The listing builds one solid part. Answer for the finished solid, in the listing's coordinates (mm). A direction names the side the tool comes from. Coordinates: 2 decimals unless noted, no trailing zeros. Order: outer loops, then holes, each group sorted by start corner. A loop starts at its lowest first (then second) coordinate and runs counter-clockwise, first axis right, second up. Notation, with made-up numbers: (-0.5, 26) -> (46.5, 26) arc R18 ccw to (46.5, 30) -> close; hole circle Ø10 at (38.5, 50). An arc over 180 degrees is marked (long way). One line per question, with ' | ' between items.
from build123d import *

# Parameters (mm, degrees)
SKETCH_1_R          = 39
EXTRUDE_1_DEPTH     = 4
SKETCH_3_R          = 37
EXTRUDE_2_DEPTH     = 8
SKETCH_4_R          = 36
EXTRUDE_3_DEPTH     = 8
SKETCH_5_W          = 3
SKETCH_5_H          = 1.5
SKETCH_7_R          = 27
CUT_EXTRUDE_1_DEPTH = 17
CHAMFER_2_SIZE      = 1
SKETCH_14_R         = 1.3
CUT_EXTRUDE_4_DEPTH = 7
CUT_EXTRUDE_START   = 7
SKETCH_16_R         = 1.3
CUT_EXTRUDE_5_DEPTH = 7
SKETCH_18_R         = 1.3
CUT_EXTRUDE_6_DEPTH = 7
CHAMFER_3_SIZE      = 1


with BuildPart() as part:
    # Sketch 1 → Бобышка-Вытянуть1 (new body)
    with BuildSketch(Plane.XY):
        Circle(SKETCH_1_R)
    extrude(amount=EXTRUDE_1_DEPTH)

    # Эскиз3 → Бобышка-Вытянуть2 (add)
    with BuildSketch(Plane(origin=(0, 0, 0), x_dir=(-1, 0, 0), z_dir=(0, 0, -1))):
        with Locations(Location((0, 0, 0), (0, 0, 180))):
            Circle(SKETCH_3_R)
    extrude(amount=EXTRUDE_2_DEPTH)

    # Эскиз4 → Бобышка-Вытянуть3 (add)
    with BuildSketch(Plane(origin=(0, 0, -8), x_dir=(-1, 0, 0), z_dir=(0, 0, -1))):
        Circle(SKETCH_4_R)
    extrude(amount=EXTRUDE_3_DEPTH)

    # Эскиз5 → Вырез-Повернуть1 (revolve, cut)
    with BuildSketch(Plane(origin=(0, 0, 0), x_dir=(0, 0, -1), z_dir=(1, 0, 0)), mode=Mode.PRIVATE) as cut_revolve_1_sk:
        with Locations((12.5, 35.25)):
            Rectangle(SKETCH_5_W, SKETCH_5_H)
    revolve(cut_revolve_1_sk.sketch.rotate(Axis((0, 0, 46.650977883), (0, 0, -1)), 90), axis=Axis((0, 0, 46.650977883), (0, 0, -1)), mode=Mode.SUBTRACT)

    # Эскиз7 → Вырез-Вытянуть1 (cut)
    with BuildSketch(Plane(origin=(0, 0, -16), x_dir=(-1, 0, 0), z_dir=(0, 0, -1))):
        Circle(SKETCH_7_R)
    extrude(amount=-CUT_EXTRUDE_1_DEPTH, mode=Mode.SUBTRACT)

    # Фаска2
    chamfer_2_edges = [part.edges().sort_by_distance(p)[0] for p in [
        (36, 0, -16),
    ]]
    chamfer(chamfer_2_edges, length=CHAMFER_2_SIZE)

    # Эскиз14 → Вырез-Вытянуть4 (cut)
    with BuildSketch(Plane(origin=(37, 0, 0), x_dir=(0, 0, -1), z_dir=(1, 0, 0))):
        with Locations((5, 0)):
            Circle(SKETCH_14_R)
    extrude(amount=-CUT_EXTRUDE_4_DEPTH, mode=Mode.SUBTRACT)

    # Эскиз16 → Вырез-Вытянуть5 (cut)
    with BuildSketch(Plane(origin=(-37, 0, 0), x_dir=(0, 0, -1), z_dir=(1, 0, 0)).offset(CUT_EXTRUDE_START)):
        with Locations((5, 0)):
            Circle(SKETCH_16_R)
    extrude(amount=-CUT_EXTRUDE_5_DEPTH, mode=Mode.SUBTRACT)

    # Эскиз18 → Вырез-Вытянуть6 (cut)
    with BuildSketch(Plane.XY.offset(4)):
        with Locations((6.5, 32.5)):
            Circle(SKETCH_18_R)
        with Locations(Location((-6.5, 32.5, 0), (0, 0, 180))):
            Circle(SKETCH_18_R)
        with Locations(Location((6.5, -32.5, 0), (0, 0, 180))):
            Circle(SKETCH_18_R)
        with Locations((-6.5, -32.5)):
            Circle(SKETCH_18_R)
    extrude(amount=-CUT_EXTRUDE_6_DEPTH, mode=Mode.SUBTRACT)

    # Фаска3
    chamfer_3_edges = [part.edges().sort_by_distance(p)[0] for p in [
        (27, 0, 1),
        (27, 0, -16),
        (-39, 0, 4),
    ]]
    chamfer(chamfer_3_edges, length=CHAMFER_3_SIZE)


solid = part.part
Item 1: Section A-A, the plane z = -9 is taken. Give the vertices of the cut face in (x, y), plus the area to 3 significant figures.
Computed values:
outline: circle Ø72 at (0, 0); hole circle Ø54 at (0, 0) | area: 1,780 mm^2
Item 2: Find the intervals of material crossed by L1, parallel to Z at x = -33, y = 0; L2, parallel to Y at x = 0, z = -6; L3, parallel to Z at x = -27, y = 26, in increasing order.
Computed values:
L1: z = -16 to -6.3, -3.7 to 4 | L2: y = -37 to -27, 27 to 37 | L3: z = 0 to 4
Item 3: Determine the mould class of faces 1 (the face through (33.5, -0.5, -6.2)), 2 (the face through (4.686, 35.694, -14.493)), 3 (the face through (0, 0, 1)), 4 (the face through (-30, 0, -5)) for opening direction X: pulls with the +X half, pulls with the -X half, needs draft (parallel to the pull), parting line crosses it, or undercut.
Computed values:
face 1: needs draft | face 2: parting line crosses it | face 3: undercut | face 4: pulls with the -X half
Item 4: Each of these flat-tipped pins is pushed along its axis until it touches: pin 1 Ø10 at (x, z) = (22.5, -9) entering from +Y; pin 2 Ø2 at (x, y) = (7, -32.5) entering from +Z; pin 3 Ø4 at (x, z) = (-22.5, -8.5) entering from +Y; pin 4 Ø2 at (x, z) = (18, -4) entering from +Y. Where does it stop, or does it pass through?
Computed values:
pin 1: stops at y = 32.55 | pin 2: stops at z = 4 | pin 3: stops at y = 30.76 | pin 4: stops at y = 32.86
Item 5: For faces 5 (the face through (8, 35.5, -8)), 6 (the face through (5.801, -33.596, 0.549)), 7 (the face through (-33.5, -0.5, -6.2)), 8 (the face through (-34.467, -1.517, -12.521)), determine the directions among +Z, -Z, +X, -X, +Y, -Y from which every point of the face is accessible in a straight line to the end or side of a thin tool.
Computed values:
face 5: -Z | face 6: +Z | face 7: -X | face 8: none
